```python
from build123d import *

# Parameters (mm, degrees)
SKETCH1_R                = 38.5
SKETCH1_R_2              = 6
BOSS_EXTRUDE1_DEPTH      = 180
BOSS_EXTRUDE2_DEPTH      = 210
BOSS_EXTRUDE2_DEPTH_BACK = 15
SKETCH1_3_R              = 6


with BuildPart() as part:
    # Sketch1 → Boss-Extrude1 (new body)
    with BuildSketch(Plane(origin=(0, 0, 0), x_dir=(0, 0, -1), z_dir=(1, 0, 0))):
        with Locations(Location((0, 0, 0), (0, 0, 180))):
            Circle(SKETCH1_R)
        with Locations(Location((0, 0, 0), (0, 0, 180))):
            Circle(SKETCH1_R_2, mode=Mode.SUBTRACT)
    extrude(amount=BOSS_EXTRUDE1_DEPTH)

    # Sketch1_3 → Boss-Extrude2 (add, two sides: drawn at the far end of the back side and taken through both)
    with BuildSketch(Plane(origin=(0, 0, 0), x_dir=(0, 0, -1), z_dir=(1, 0, 0)).offset(-BOSS_EXTRUDE2_DEPTH_BACK)):
        Circle(SKETCH1_3_R)
    extrude(amount=BOSS_EXTRUDE2_DEPTH + BOSS_EXTRUDE2_DEPTH_BACK)


solid = part.part
```
The model under review builds one solid part; all positions refer to its coordinate system, in mm. A direction names the side the tool comes from. Round coordinates to 2 decimals unless told otherwise and drop trailing zeros. Write each loop counter-clockwise with the first axis right and the second up, starting at its lowest first coordinate (ties: lowest second). Pieces come first, ordered by that corner, then holes. Notation, with made-up numbers: (11, 51.5) - (30, 51.5) arc R23 cw to (30, 85.5) - close; hole circle Ø11 at (-36, 37). An arc over 180 degrees is marked (long way). Use one line per item in the form item = value.
Q1. Consider section C-C (x = 86). State the section outline as (y, z) points.
Answer key:
outline = circle Ø77 at (0, 0)
Q2. Consider section D-D (x = 189.5). State the section outline as (y, z) points.
Answer key:
outline = circle Ø12 at (0, 0)
Q3. Tool access review of faces 1 (the cylindrical face through (-8, 0, 6)), 2 (the cylindrical face through (195, 0, 6)), 3 (the cylindrical face through (88.74, 23.43, -30.55)): name each direction out of +Z, -Z, +X, -X, +Y, -Y from which nothing blocks a thin tool from reaching the whole face with its end or side.
Answer key:
face_1 = -X
face_2 = +X
face_3 = +X, -X
Q4. For line 1 (X direction, y = 2.5, z = 31); line 2 (Z direction, x = 122, y = -30); line 3 (Z direction, x = 20, y = 16.5), list the stretches that pass through material, from the lowest coordinate up. Write a range as [from, to].
Answer key:
line_1 = [0, 180]
line_2 = [-24.13, 24.13]
line_3 = [-34.79, 34.79]
Q5. Insertion check: pin 1 Ø8 at (x, y) = (108, 10.5) entering from -Z; pin 2 Ø12 at (y, z) = (19, -1) entering from +X; pin 3 Ø10 at (x, y) = (69, -17) entering from +Z. Each pin has a flat end and moves straight along its axis. Give the tip position at first contact, or say it passes through.
Answer key:
pin_1 = -37.95
pin_2 = 180
pin_3 = 36.58
Q6. Consider section A-A (z = 0). State the section outline as (x, y) points.
Answer key:
outline = (-15, -6) - (0, -6) - (0, -38.5) - (180, -38.5) - (180, -6) - (210, -6) - (210, 6) - (180, 6) - (180, 38.5) - (0, 38.5) - (0, 6) - (-15, 6) - close
